from build123d import *
from OCP.BRepFilletAPI import BRepFilletAPI_MakeFillet

# Parameters (mm, degrees)
SKETCH1_W               = 33
SKETCH1_H               = 40
BOSS_EXTRUDE1_DEPTH     = 1
SKETCH3_R               = 1.2
BOSS_EXTRUDE2_DEPTH     = 3
BOSS_EXTRUDE3_START     = -3
SKETCH4_R               = 1.2
BOSS_EXTRUDE3_DEPTH     = 3
CUT_EXTRUDE1_DEPTH      = 30.550803712
CUT_EXTRUDE1_DEPTH_BACK = 30.550803712
SKETCH6_R               = 1.5
SKETCH6_W               = 18
SKETCH6_H               = 3
FILLET4_R1              = 2
FILLET4_R2              = 1
CUT_EXTRUDE2_DEPTH      = 27
FILLET5_R               = 0.5


with BuildPart() as part:
    # Sketch1 → Boss-Extrude1 (new, symmetric)
    with BuildSketch(Plane.XY):
        Rectangle(SKETCH1_W, SKETCH1_H)
    extrude(amount=BOSS_EXTRUDE1_DEPTH, both=True)

    # Sketch3 → Boss-Extrude2 (add)
    with BuildSketch(Plane(origin=(16.5, 0, 0), x_dir=(0, 0, -1), z_dir=(1, 0, 0))):
        with BuildLine():
            Line((-1, -20), (-1, -21))
            ThreePointArc((-1, -21), (4.449489743, -22.732050808), (1, -18.171572875))
            Line((1, -18.171572875), (-1, -20))
        make_face()
        with Locations((2, -21)):
            Circle(SKETCH3_R, mode=Mode.SUBTRACT)
    extrude(amount=-BOSS_EXTRUDE2_DEPTH)

    # Sketch4 → Boss-Extrude3 (add)
    with BuildSketch(Plane.ZY.offset(16.5).offset(BOSS_EXTRUDE3_START)):
        with BuildLine():
            Line((1, -20), (1, -21))
            ThreePointArc((1, -21), (-4.449489743, -22.732050808), (-1, -18.171572875))
            Line((-1, -18.171572875), (1, -20))
        make_face()
        with Locations(Location((-2, -21, 0), (0, 0, 180))):
            Circle(SKETCH4_R, mode=Mode.SUBTRACT)
    extrude(amount=BOSS_EXTRUDE3_DEPTH)

    # Sketch6 → Cut-Extrude1 (cut, two sides: drawn at the far end of the back side and taken through both)
    with BuildSketch(Plane.XY.offset(-CUT_EXTRUDE1_DEPTH_BACK)):
        with Locations((-12, 12.25)):
            Circle(SKETCH6_R)
        with Locations((12, 12.25)):
            Circle(SKETCH6_R)
        with Locations((12, -12.25)):
            Circle(SKETCH6_R)
        with Locations((-12, -12.25)):
            Circle(SKETCH6_R)
        with Locations((0, 16.75)):
            Rectangle(SKETCH6_W, SKETCH6_H)
    extrude(amount=CUT_EXTRUDE1_DEPTH + CUT_EXTRUDE1_DEPTH_BACK, mode=Mode.SUBTRACT)

    # Fillet4: one fillet with a radius per group of edges: ONE call of the kernel's fillet builder (fillet() takes one radius for all edges)
    fillet4_edges_1 = [part.edges().sort_by_distance(p)[0] for p in [
        (16.5, 20, 0),
        (15, -18.171572875, -1),
        (-15, -18.171572875, -1),
    ]]
    fillet4_edges_2 = [part.edges().sort_by_distance(p)[0] for p in [
        (-16.5, 20, 0),
        (-9, 18.25, 0),
        (-9, 15.25, 0),
        (9, 18.25, 0),
        (9, 15.25, 0),
    ]]
    fillet4 = BRepFilletAPI_MakeFillet(part.part.solid().wrapped)
    for e in fillet4_edges_1:
        fillet4.Add(FILLET4_R1, e.wrapped)
    for e in fillet4_edges_2:
        fillet4.Add(FILLET4_R2, e.wrapped)
    add(Compound.cast(fillet4.Shape()), mode=Mode.REPLACE)

    # Sketch8 → Cut-Extrude2 (cut)
    with BuildSketch(Plane.ZY.offset(-13.5)):
        Polygon((-1, -16.101020514), (1, -20), (-1, -20), align=None)
    extrude(amount=CUT_EXTRUDE2_DEPTH, mode=Mode.SUBTRACT)

    # Fillet5
    fillet5_edges = [part.edges().sort_by_distance(p)[0] for p in [
        (0, -20, 1),
    ]]
    fillet(fillet5_edges, radius=FILLET5_R)


solid = part.part
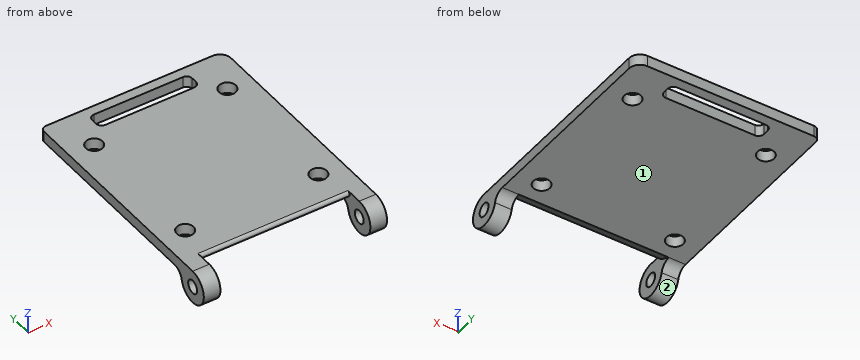
Build history of the part. All positions in model axes, mm. Face numbers are marked on the shaded views. A direction names the side the tool comes from. Round coordinates to 2 decimals unless told otherwise and drop trailing zeros. Loops run counter-clockwise (first coordinate to the right, second up) from the corner with the lowest first, then second, coordinate; pieces in that order, holes last. Notation, with made-up numbers: (77, -2) -> (128, -2) arc R13 cw to (128, 11) -> close; hole circle Ø10 at (23, 17.5). An arc over 180 degrees is marked (long way). One line per item, written item: value. Start each with the question number.
Q1. Cut at C-C on x = 4.5. List the corners of the cut face in (y, z), plus the area to 3 significant figures.
Q2. Cut at A-A on x = -12. List the corners of the cut face in (y, z).
Q3. 3-axis set-ups, long thin cutter, end or side, ignore diameter. For the marked faces 1 and 2: which of +Z, -Z, +X, -X, +Y, -Y reach the whole face in a straight line?
Q4. Probe line 1 along Y through (x, z) = (-12, 0); line 2 along Y through (x, z) = (12, 0.55); line 3 along Z through (x, y) = (-6, 1). List the from-to ranges inside material, lowest first.
Q5. Cut at D-D on z = -2. List the corners of the cut face in (x, y).
Q6. Drop flat-ended pins along their axis: pin 1 Ø5 at (x, y) = (3.5, 14.5) entering from -Z; pin 2 Ø4 at (x, y) = (12, -12.25) entering from +Z; pin 3 Ø2 at (x, z) = (-1.5, -0.5) entering from -Y. Give the stop position or say it passes through.
Q7. Cut at B-B on y = 12.25. List the corners of the cut face in (x, z).
Computed:
1. outline: (-18.16, 0.06) -> (-16.1, -1) -> (15.25, -1) -> (15.25, 1) -> (-17.93, 1) arc R0.5 ccw to start; (18.25, -1) -> (20, -1) -> (20, 1) -> (18.25, 1) -> close
1. area: 69.4 mm²
2. outline: (-18.16, 0.06) -> (-16.1, -1) -> (-13.75, -1) -> (-13.75, 1) -> (-17.93, 1) arc R0.5 ccw to start; (-10.75, -1) -> (10.75, -1) -> (10.75, 1) -> (-10.75, 1) -> close; (13.75, -1) -> (20, -1) -> (20, 1) -> (13.75, 1) -> close
3. face 1: -Z, +X, -X, +Y
3. face 2: +X, -X
4. line 1: -18.05 to -13.75, -10.75 to 10.75, 13.75 to 20
4. line 2: -18.43 to -13.75, -10.75 to 10.75, 13.75 to 20
4. line 3: -1 to 1
5. outline: (-16.5, -24) -> (-13.5, -24) -> (-13.5, -22.2) -> (-16.5, -22.2) -> close; (-16.5, -19.8) -> (-13.5, -19.8) -> (-13.5, -17.83) -> (-16.5, -17.83) -> close; (13.5, -24) -> (16.5, -24) -> (16.5, -22.2) -> (13.5, -22.2) -> close; (13.5, -19.8) -> (16.5, -19.8) -> (16.5, -17.83) -> (13.5, -17.83) -> close
6. pin 1: z = -1
6. pin 2: z = 1
6. pin 3: y = -18.43
7. outline: (-16.5, -1) -> (-13.5, -1) -> (-13.5, 1) -> (-16.5, 1) -> close; (-10.5, -1) -> (10.5, -1) -> (10.5, 1) -> (-10.5, 1) -> close; (13.5, -1) -> (16.5, -1) -> (16.5, 1) -> (13.5, 1) -> close
